CAD build for the part. Positions are in the model's coordinates, mm. Face numbers are marked on the shaded views. A direction names the side the tool comes from. Give positions to 0.01 mm unless a question says otherwise; leave off trailing zeros. Order: outer loops, then holes, each group sorted by start corner. A loop starts at its lowest first (then second) coordinate and runs counter-clockwise, first axis right, second up.
from build123d import *

# Parameters (mm, degrees)
BASE_FLANGE1_DEPTH           = 31.75
SKETCH6_R                    = 25.4
CUT_EXTRUDE1_DEPTH           = 150.764450471
FILLET1_R                    = 2.54
CUT_EXTRUDE2_DEPTH           = 82.875610685
F_7_0_201_DIAMETER_HOLE1_D   = 5.1054
F_25_0_1495_DIAMETER_HOLE1_D = 3.7973


# Sheet-metal steps are written as plain solids
with BuildPart() as part:
    # Sketch1 → Base-Flange1 (new, symmetric)
    with BuildSketch(Plane(origin=(0, 0, 0), x_dir=(-1, 0, 0), z_dir=(0, 1, 0))):
        with BuildLine():
            Line((9.525, -73.025), (9.525, 68.453))
            ThreePointArc((9.525, 68.453), (8.185892204, 71.685892204), (4.953, 73.025))
            Line((4.953, 73.025), (-9.525, 73.025))
            Line((-9.525, 73.025), (-9.525, 70.739))
            Line((-9.525, 70.739), (4.953, 70.739))
            ThreePointArc((4.953, 70.739), (6.569446102, 70.069446102), (7.239, 68.453))
            Line((7.239, 68.453), (7.239, -73.025))
            Line((7.239, -73.025), (9.525, -73.025))
        make_face()
    extrude(amount=BASE_FLANGE1_DEPTH, both=True)

    # Sketch6 → Cut-Extrude1 (cut, through all)
    with BuildSketch(Plane.XY.offset(73.025)):
        with Locations((22.225, 0)):
            Circle(SKETCH6_R)
    extrude(amount=-CUT_EXTRUDE1_DEPTH, mode=Mode.SUBTRACT)

    # Fillet1
    fillet1_edges = [part.edges().sort_by_distance(p)[0] for p in [
        (9.525, 31.75, 71.882),
        (9.525, -31.75, 71.882),
    ]]
    fillet(fillet1_edges, radius=FILLET1_R)

    # Sketch7 → Cut-Extrude2 (cut, through all)
    with BuildSketch(Plane(origin=(-9.525, 0, 0), x_dir=(0, -1, 0), z_dir=(-1, 0, 0))):
        with BuildLine():
            Line((-31.75, -41.275), (-31.75, -92.075))
            Line((-31.75, -92.075), (31.75, -92.075))
            Line((31.75, -92.075), (31.75, -41.275))
            ThreePointArc((31.75, -41.275), (0, -73.025), (-31.75, -41.275))
        make_face()
    extrude(amount=-CUT_EXTRUDE2_DEPTH, mode=Mode.SUBTRACT)

    # #7 (0.201) Diameter Hole1 (through all)
    with Locations(Plane.ZY.offset(9.525)):
        with Locations((-41.275, 0)):
            Hole(F_7_0_201_DIAMETER_HOLE1_D / 2)

    # #25 (0.1495) Diameter Hole1 (through all)
    with Locations(Plane.XY.offset(73.025)):
        with Locations((3.175, 25.4), (3.175, -25.4)):
            Hole(F_25_0_1495_DIAMETER_HOLE1_D / 2)


solid = part.part
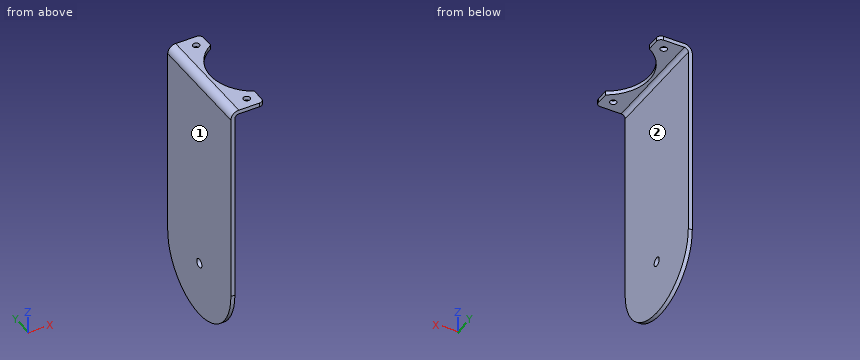
1. Saw through at D-D on y = -25.4. Give the cut face in (x, z) (3 decimals).
2. 3-axis set-ups, long thin cutter, end or side, ignore diameter. For the marked faces 1 and 2: which of +Z, -Z, +X, -X, +Y, -Y reach the whole face in a straight line?
3. Saw through at A-A on y = 0. Give the cut face in (x, z) (3 decimals), plus the area to 3 significant figures.
4. Wall check: line 1 (Z direction, x = 1.25, y = -20) (3 decimals); line 2 (X direction, y = 29, z = -8) (3 decimals); line 3 (X direction, y = 25, z = 71) (3 decimals). Give the ranges that are in metal, low to high.
5. Saw through at C-C on z = 7. Give the cut face in (x, y) (3 decimals).
6. Pin check, flat tips, straight feed: P1, Ø4.5, axis at x = 2, y = 10.5, coming from the -Z side; P2, Ø10, axis at y = -24, z = 13, coming from the +X side; P3, Ø5, axis at x = 1.5, y = 14, coming from the -Z side. Stop position of each tip, or through.
7. Saw through at B-B on y = -15. Give the cut face in (x, z) (3 decimals), plus the area to 3 significant figures.
Reported:
1. outline: (-9.525, -60.325) - (-7.239, -60.325) - (-7.239, 68.453) arc R2.286 cw to (-4.953, 70.739) - (1.276, 70.739) - (1.276, 73.025) - (-4.953, 73.025) arc R4.572 ccw to (-9.525, 68.453) - close; (5.074, 70.739) - (9.525, 70.739) - (9.525, 73.025) - (5.074, 73.025) - close
2. face 1: +Z, -Z, -X, +Y, -Y
2. face 2: -Z, +X, +Y, -Y
3. outline: (-9.525, -73.025) - (-7.239, -73.025) - (-7.239, -43.828) - (-9.525, -43.828) - close; (-9.525, -38.722) - (-7.239, -38.722) - (-7.239, 68.453) arc R2.286 cw to (-4.953, 70.739) - (-3.175, 70.739) - (-3.175, 73.025) - (-4.953, 73.025) arc R4.572 ccw to (-9.525, 68.453) - close
3. area: 328 mm2
4. line 1: z = 70.739 to 73.025
4. line 2: x = -9.525 to -7.239
4. line 3: x = -8.75 to 1.319, 5.031 to 9.525
5. outline: (-9.525, -31.75) - (-7.239, -31.75) - (-7.239, 31.75) - (-9.525, 31.75) - close
6. P1: passes through
6. P2: stops at x = -7.24
6. P3: stops at z = 70.74
7. outline: (-9.525, -69.258) - (-7.239, -69.258) - (-7.239, 68.453) arc R2.286 cw to (-4.953, 70.739) - (1.727, 70.739) - (1.727, 73.025) - (-4.953, 73.025) arc R4.572 ccw to (-9.525, 68.453) - close
7. area: 342 mm2
